```python
from build123d import *

# Parameters (mm, degrees)
SKETCH1_W             = 50
SKETCH1_H             = 10
BOSS_EXTRUDE1_DEPTH   = 100
SKETCH2_W             = 10
SKETCH2_H             = 100
BOSS_EXTRUDE2_DEPTH   = 38.1
SKETCH3_W             = 100
SKETCH3_H             = 10
BOSS_EXTRUDE3_DEPTH   = 25.4
M5X0_8_TAPPED_HOLE1_D = 5
M5X0_8_TAPPED_HOLE2_D = 5


with BuildPart() as part:
    # Sketch1 → Boss-Extrude1 (new body)
    with BuildSketch(Plane.XY):
        Rectangle(SKETCH1_W, SKETCH1_H)
    extrude(amount=BOSS_EXTRUDE1_DEPTH)

    # Sketch2 → Boss-Extrude2 (add)
    with BuildSketch(Plane.XZ.offset(5)):
        with Locations((-20, 50)):
            Rectangle(SKETCH2_W, SKETCH2_H)
    extrude(amount=BOSS_EXTRUDE2_DEPTH)

    # Sketch3 → Boss-Extrude3 (add)
    with BuildSketch(Plane.ZY.offset(25)):
        with Locations((50, -38.1)):
            Rectangle(SKETCH3_W, SKETCH3_H)
    extrude(amount=BOSS_EXTRUDE3_DEPTH)

    # M5x0.8 Tapped Hole1 (through all)
    with Locations(Plane(origin=(0, 5, 0), x_dir=(1, 0, 0), z_dir=(0, 1, 0))):
        with Locations((12.3, -75), (12.3, -25)):
            Hole(M5X0_8_TAPPED_HOLE1_D / 2)

    # M5x0.8 Tapped Hole2 (through all)
    with Locations(Plane(origin=(-15, 0, 0), x_dir=(0, 0, -1), z_dir=(1, 0, 0))):
        with Locations((-27, -8.1), (-73, -26.1), (-27, -26.1), (-73, -8.1)):
            Hole(M5X0_8_TAPPED_HOLE2_D / 2)


solid = part.part
```
Geometry check sheet. Reference: the model listing, model coordinates, mm. A direction names the side the tool comes from. Give positions to 0.01 mm unless a question says otherwise; leave off trailing zeros. Order: outer loops, then holes, each group sorted by start corner. A loop starts at its lowest first (then second) coordinate and runs counter-clockwise, first axis right, second up. Notation, with made-up numbers: (87, -33.75) - (132, -33.75) arc R16 ccw to (132, -24.75) - close; hole circle Ø7 at (4, -6.75). An arc over 180 degrees is marked (long way). Answer in a Markdown table with one row per item. Add a question column.
Q1. Cross-section at B-B, the plane y = -26.1. Enter the section's corners in (x, z), then the cut area to 3 significant figures.
Q2. Cross-section at C-C, the plane x = -18. Enter the section's corners in (y, z), then the cut area to 3 significant figures.
Q3. Cross-section at D-D, the plane z = 15. Enter the section's corners in (x, y).
Q4. Tool access check on faces 1 (the flat face through (-15, -24, 49)), 2 (the cylindrical face through (-20.07, -6.41, 25.16)), 3 (the flat face through (-38, -33.1, 49)). Record the directions out of +Z, -Z, +X, -X, +Y, -Y that give a thin tool (end or side, any length) a straight path to the whole face; none if there is none.
Q5. Mould release check, pull along Z, two halves, no side actions. Record for faces 4 (the cylindrical face through (12.84, -0.07, 77.44)), 5 (the flat face through (-32, -43.1, 49)), 6 (the flat face through (-18, -17, 0)), 7 (the flat face through (-18, -17, 100)): pulls with the +Z half, pulls with the -Z half, needs draft (parallel to the pull), parting line crosses it, or undercut.
Q6. Gauge pin test, flat ends, axial feed: pin 1 (3 mm diameter, centred on y = -30, z = 47.5, fed in from -X); pin 2 (10 mm diameter, centred on y = -17.5, z = 66.5, fed in from +X). Record the tip position at first contact, or that the pin passes through.
Q7. Material ranges on probe 1 along Z at (x, y) = (12.3, -2.25); probe 2 along Y at (x, z) = (-21, 27); probe 3 along X at (y, z) = (1, 75), recorded low to high. Write a range as from..to.
Q8. Cross-section at A-A, the plane x = 12.3. Enter the section's corners in (y, z).
Check values:
| question | item | result |
|---|---|---|
| 1 | outline | (-25, 0) - (-15, 0) - (-15, 24.5) - (-25, 24.5) - close; (-25, 29.5) - (-15, 29.5) - (-15, 70.5) - (-25, 70.5) - close; (-25, 75.5) - (-15, 75.5) - (-15, 100) - (-25, 100) - close |
| 1 | area | 900 mm^2 |
| 2 | outline | (-43.1, 0) - (5, 0) - (5, 100) - (-43.1, 100) - close; hole circle Ø5 at (-26.1, 27); hole circle Ø5 at (-26.1, 73); hole circle Ø5 at (-8.1, 27); hole circle Ø5 at (-8.1, 73) |
| 2 | area | 4,730 mm^2 |
| 3 | outline | (-50.4, -43.1) - (-15, -43.1) - (-15, -5) - (25, -5) - (25, 5) - (-25, 5) - (-25, -33.1) - (-50.4, -33.1) - close |
| 4 | face 1 | +Z, -Z, +X, -Y |
| 4 | face 2 | +X, -X |
| 4 | face 3 | +Z, -Z, -X, +Y |
| 5 | face 4 | undercut |
| 5 | face 5 | needs draft |
| 5 | face 6 | pulls with the -Z half |
| 5 | face 7 | pulls with the +Z half |
| 6 | pin 1 | stops at x = -25 |
| 6 | pin 2 | stops at x = -15 |
| 7 | probe 1 | z = 0..22.5, 27.5..72.5, 77.5..100 |
| 7 | probe 2 | y = -43.1..-28.6, -23.6..-10.6, -5.6..5 |
| 7 | probe 3 | x = -25..9.8, 14.8..25 |
| 8 | outline | (-5, 0) - (5, 0) - (5, 22.5) - (-5, 22.5) - close; (-5, 27.5) - (5, 27.5) - (5, 72.5) - (-5, 72.5) - close; (-5, 77.5) - (5, 77.5) - (5, 100) - (-5, 100) - close |
